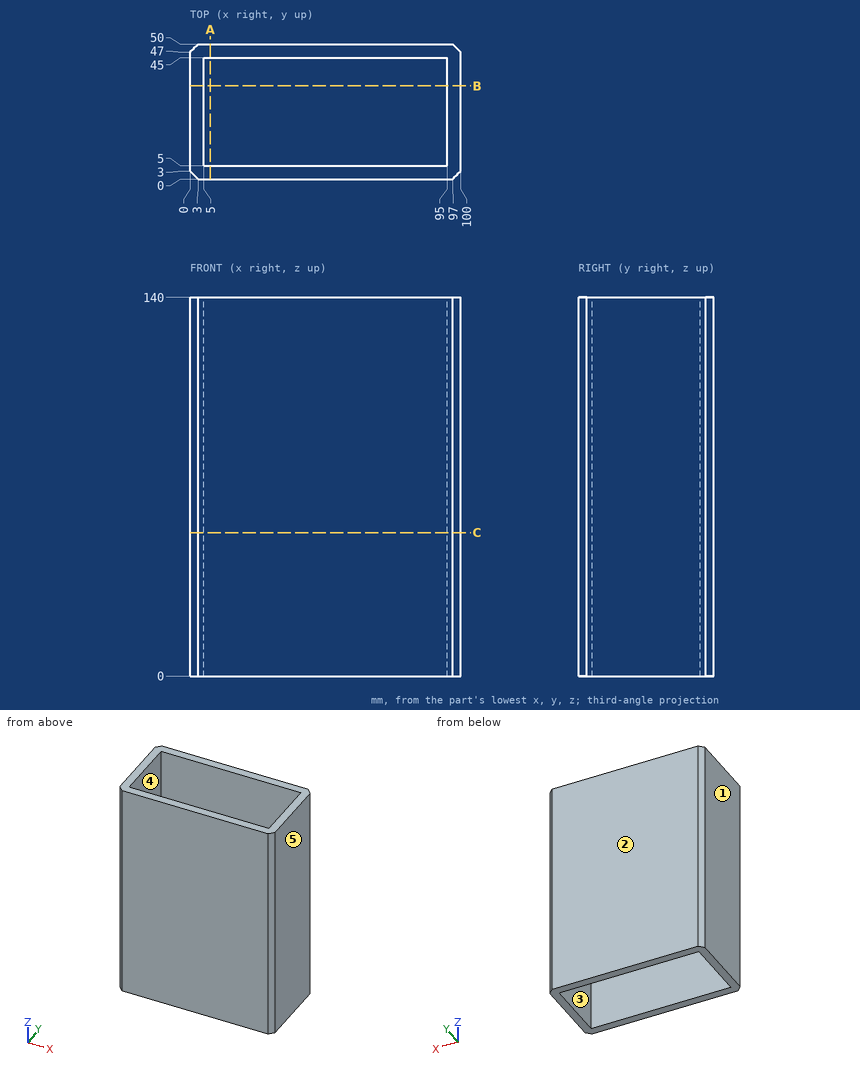
Part print with two shaded views. Sizes in mm from the minimum x, y, z corner. A direction names the side the tool comes from. Give positions to 0.01 mm unless a question says otherwise; leave off trailing zeros. Order: outer loops, then holes, each group sorted by start corner. A loop starts at its lowest first (then second) coordinate and runs counter-clockwise, first axis right, second up.
(1) Saw through at B-B, the plane y = 34.5. Give the cut face in (x, z), then the cut area to 3 significant figures.
(2) Tool access for the marked faces 4 and 5: list every direction of +Z, -Z, +X, -X, +Y, -Y with a clear straight run to the whole face (end or side of a thin tool).
(3) Mould opens along Y. For the marked faces 1, 2 and 3 say: released by +Y, released by -Y, zero draft, split by the parting line, or undercut.
(4) Drill centre lines: L1, parallel to X at y = 25.5, z = 110; L2, parallel to Y at x = 10.5, z = 60. Where is each one in solid material? Low to high.
(5) Saw through at C-C, the plane z = 53. Give the cut face in (x, y), then the cut area to 3 significant figures.
(6) Saw through at A-A, the plane x = 7.5. Give the cut face in (y, z), then the cut area to 3 significant figures.
Results found:
1. outline: (0, 0) - (5, 0) - (5, 140) - (0, 140) - close; (95, 0) - (100, 0) - (100, 140) - (95, 140) - close
1. area: 1,400 mm2
2. face 4: +Z, -Z
2. face 5: +Z, -Z, +X, +Y, -Y
3. face 1: zero draft
3. face 2: released by +Y
3. face 3: undercut
4. L1: x = 0 to 5, 95 to 100
4. L2: y = 0 to 5, 45 to 50
5. outline: (0, 3) - (3, 0) - (97, 0) - (100, 3) - (100, 47) - (97, 50) - (3, 50) - (0, 47) - close; hole (5, 5) - (95, 5) - (95, 45) - (5, 45) - close
5. area: 1,380 mm2
6. outline: (0, 0) - (5, 0) - (5, 140) - (0, 140) - close; (45, 0) - (50, 0) - (50, 140) - (45, 140) - close
6. area: 1,400 mm2
